For this review, take the finished solid that the model builds, in its own axes (mm). A direction names the side the tool comes from. Round coordinates to 2 decimals unless told otherwise and drop trailing zeros. Order: outer loops, then holes, each group sorted by start corner. A loop starts at its lowest first (then second) coordinate and runs counter-clockwise, first axis right, second up. Notation, with made-up numbers: (2.25, 53) -> (9.25, 53) arc R26 cw to (9.25, 81) -> close; hole circle Ø6 at (66.5, 28). An arc over 180 degrees is marked (long way). Answer in a Markdown table with one row per item.
```python
from build123d import *

# Parameters (mm, degrees)
F0_R     = 10
F1_DEPTH = 15
F3_DEPTH = 10
F5_DEPTH = 10


with BuildPart() as f1:
    # F0 (on Top) → F1 (new body)
    with BuildSketch(Plane.XY):
        Circle(F0_R)
    extrude(amount=F1_DEPTH)

    # F2 (on face) → F3 (cut)
    with BuildSketch(Plane(origin=(0, 0, 0), x_dir=(1, 0, 0), z_dir=(0, 0, -1))):
        with BuildLine():
            Line((-2.516446, -3.3), (2.516446, -3.3))
            ThreePointArc((2.516446, -3.3), (0, 4.15), (-2.516446, -3.3))
        make_face()
    extrude(amount=-F3_DEPTH, mode=Mode.SUBTRACT)

    # F4 (on face) → F5 (join)
    with BuildSketch(Plane.XY.offset(15)):
        with BuildLine():
            Line((1.615549, 1), (-1.615549, 1))
            ThreePointArc((-1.615549, 1), (0, -1.9), (1.615549, 1))
        make_face()
    extrude(amount=F5_DEPTH)


solid = f1.part
```
Q1. Clearance check with flat-ended pins moving along their axes: pin 1 Ø4 at (y, z) = (3.5, 8.5) entering from +X; pin 2 Ø6 at (y, z) = (-7, 15.5) entering from -X; pin 3 Ø3.5 at (x, y) = (0.5, -2) entering from -Z. State where each tip first meets the part, or that it passes through.
Answer key:
| item | result |
|---|---|
| pin 1 | stops at x = 9.89 |
| pin 2 | stops at x = -9.15 |
| pin 3 | stops at z = 10 |
Q2. Take a section at C-C, the plane y = 2. Write out the cut boundary in (x, z), then the cut area to 3 significant figures.
Answer key:
| item | result |
|---|---|
| outline | (-9.8, 0) -> (-3.64, 0) -> (-3.64, 10) -> (3.64, 10) -> (3.64, 0) -> (9.8, 0) -> (9.8, 15) -> (-9.8, 15) -> close |
| area | 221 mm^2 |
Q3. Take a section at D-D, the plane x = -8. Write out the cut boundary in (y, z), then the cut area to 3 significant figures.
Answer key:
| item | result |
|---|---|
| outline | (-6, 0) -> (6, 0) -> (6, 15) -> (-6, 15) -> close |
| area | 180 mm^2 |
Q4. Take a section at A-A, the plane x = 0. Write out the cut boundary in (y, z).
Answer key:
| item | result |
|---|---|
| outline | (-10, 0) -> (-4.15, 0) -> (-4.15, 10) -> (3.3, 10) -> (3.3, 0) -> (10, 0) -> (10, 15) -> (1, 15) -> (1, 25) -> (-1.9, 25) -> (-1.9, 15) -> (-10, 15) -> close |
Q5. Take a section at B-B, the plane z = 11. Write out the cut boundary in (x, y), then the cut area to 3 significant figures.
Answer key:
| item | result |
|---|---|
| outline | circle Ø20 at (0, 0) |
| area | 314 mm^2 |
Q6. To check wall thickness, follow probe 1 along X at (y, z) = (-0.25, 8); probe 2 along Y at (x, z) = (0, 4.75); probe 3 along Z at (x, y) = (7.5, -5). State the ranges of each line that lie inside material, in increasing order.
Answer key:
| item | result |
|---|---|
| probe 1 | x = -10 to -4.14, 4.14 to 10 |
| probe 2 | y = -10 to -4.15, 3.3 to 10 |
| probe 3 | z = 0 to 15 |
Q7. Tool access review of faces 1 (the face through (-0.1, -4.3, 0)), 2 (the face through (0, 1, 20)), 3 (the face through (0, 3.3, 5)): name each direction out of +Z, -Z, +X, -X, +Y, -Y from which nothing blocks a thin tool from reaching the whole face with its end or side.
Answer key:
| item | result |
|---|---|
| face 1 | -Z, +X, -X, +Y, -Y |
| face 2 | +Z, +X, -X, +Y |
| face 3 | -Z |
Q8. The part is to be moulded in two halves that separate along Y. For faces 4 (the face through (0.145, -4.147, 4.93)), 5 (the face through (0, 0, 25)), 6 (the face through (-0.06, -1.9, 19.93)), say which applies: +Y half, -Y half, draft (parallel to the pull), parting line (faces both ways), or undercut.
Answer key:
| item | result |
|---|---|
| face 4 | undercut |
| face 5 | draft |
| face 6 | parting line |
